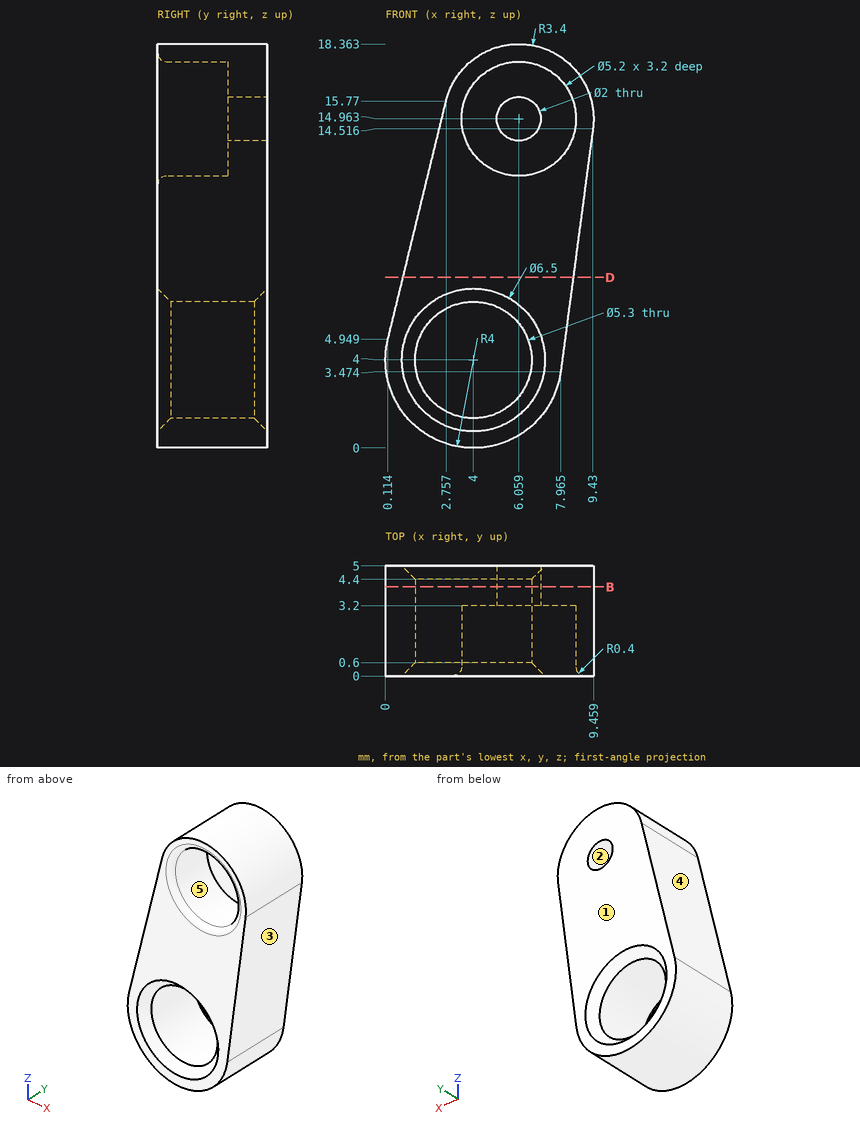
Geometry: see drawing. Coordinates: mm, zero at the bounding-box minimum. A direction names the side the tool comes from. Give positions to 0.01 mm unless a question says otherwise; leave off trailing zeros. Order: outer loops, then holes, each group sorted by start corner. A loop starts at its lowest first (then second) coordinate and runs counter-clockwise, first axis right, second up. Notation, with made-up numbers: (-19, 59) - (-3, 59) arc R16 ccw to (-3, 69) - close; hole circle Ø3 at (-35, 57). An arc over 180 degrees is marked (long way). Use CSV: the item, a comma, the result in double quotes.
1. Access query for the marked faces 4 and 5. Directions: +Z, -Z, +X, -X, +Y, -Y. A direction counts if a zero-diameter tool reaches every point of the face in a straight line with its end or side. Return the directions, or none.
Answers below:
face 4,"+Z, -X, +Y, -Y"
face 5,"-Y"
2. Material intervals for line 1 along Z through (x, y) = (5, 0.45) (1 decimal); line 2 along Z through (x, y) = (4.75, 3.05) (1 decimal); line 3 along Z through (x, y) = (5, 4.25) (1 decimal), sorted ascending. Write a range as from..to.
Answers below:
line 1,"0.1..1.4, 6.6..12.6, 17.3..18.2"
line 2,"0.1..1.5, 6.5..12.7, 17.2..18.1"
line 3,"0.1..1.5, 6.5..18.2"
3. Section query B-B (y = 4.05). Give the number of separate pieces and of enclosed holes in the cut face, plus the area to 3 significant figures.
Answers below:
separate pieces,"1"
enclosed holes,"2"
area,"101 mm2"
4. Contact query for a flat-ended pin moving along its axis: pin 1 (1.6 mm diameter, centred on x = 7, z = 16, fed in from -Y). Output: stop coordinate, or through.
Answers below:
pin 1,"y = 3.2"
5. Mould query, pull axis Z, two halves, no side actions, for the marked faces 1, 2 and 3. Classes: +Z half, -Z half, draft (parallel to the pull), parting line (faces both ways), or undercut.
Answers below:
face 1,"draft"
face 2,"undercut"
face 3,"-Z half"
6. Section query D-D (z = 7.75). Output: boundary loops of the cut face in (x, y).
Answers below:
outline,"(0.8, 0) - (8.53, 0) - (8.53, 5) - (0.8, 5) - close"
